Source: CAD feature listing. Evaluate the final solid. Frame: model axes, mm. Face numbers are marked on the shaded views. A direction names the side the tool comes from. Give positions to 0.01 mm unless a question says otherwise; leave off trailing zeros. Write each loop counter-clockwise with the first axis right and the second up, starting at its lowest first coordinate (ties: lowest second). Pieces come first, ordered by that corner, then holes. Notation, with made-up numbers: M 82,-35 L 105,-35 A28 cw 105,3 Z; hole C 9.25,12 d4. An arc over 180 degrees is marked long. Return JSON: item names as keys, results as strings.
Autodesk Inventor part; units mm, degrees
ref_plane "YZ Plane" through (0, 0, 0) normal (1, 0, 0) x (0, 1, 0)
ref_plane "XZ Plane" through (0, 0, 0) normal (0, 1, 0) x (-1, 0, 0)
ref_plane "XY Plane" through (0, 0, 0) normal (0, 0, 1) x (1, 0, 0)
sketch "Sketch1" plane through (0, 0, 0) normal (0, 1, 0) x (-1, 0, 0)
  line L0 (-6.35, 12.7) -> (-6.35, -12.7)
  line L1 (-6.35, -12.7) -> (6.35, -12.7)
  line L2 (6.35, -12.7) -> (6.35, 12.7)
  line L3 (6.35, 12.7) -> (-6.35, 12.7)
  line L4 (-6.35, 12.7) -> (6.35, -12.7) construction
  line L5 (-6.35, -12.7) -> (6.35, 12.7) construction
  line L6 (-6.35, 12.7) -> (19.05, 12.7) construction
  point P0 (0, 0)
  dimension "d0" = 25.4
  dimension "d1" = 90
  dimension "d2" = 12.7
extrude "Baseplate" add sketch "Sketch1" against normal blind 3.175
sketch "Sketch2" plane through (0, -3.175, 0) normal (0, -1, 0) x (1, 0, 0)
  circle A0 centre (3.175, -9.525) radius 1.143
  circle A1 centre (-3.175, 0) radius 1.143
  circle A2 centre (0, 8.5298) radius 1.5
  line L0 (-4.318, -8.382) -> (-2.032, -8.382)
  line L1 (-2.032, -8.382) -> (-2.032, -10.668)
  line L2 (-2.032, -10.668) -> (-4.318, -10.668)
  line L3 (-4.318, -10.668) -> (-4.318, -8.382)
  line L4 (-4.318, -8.382) -> (-2.032, -10.668) construction
  line L5 (-2.032, -8.382) -> (-4.318, -10.668) construction
  point P0 (0, 0)
  point P1 (-3.175, -9.525)
  dimension "d5" = 2.286
  dimension "d6" = 2.286
  dimension "d7" = 3
  dimension "d8" = 2.286
extrude "BoltHole" cut sketch "Sketch2" against normal blind 3.175 contours A2
extrude "Extrusion3" add sketch "Sketch2" along normal blind 3.175 contours A0 | A1 | L0 L1 L2 L3
sketch "Sketch3" plane through (0, -6.35, 0) normal (0, -1, 0) x (1, 0, 0)
  line L0 (-2.032, -11.1125) -> (-4.318, -11.1125)
  line L1 (-4.318, -11.1125) -> (-4.318, -7.9375)
  line L2 (-4.318, -7.9375) -> (-2.032, -7.9375)
  line L3 (-2.032, -7.9375) -> (-2.032, -11.1125)
  line L4 (-2.032, -11.1125) -> (-4.318, -7.9375) construction
  line L5 (-4.318, -11.1125) -> (-2.032, -7.9375) construction
  circle A0 centre (-3.175, 0) radius 1.143
  circle A1 centre (-3.175, 0) radius 1.5875
  circle A2 centre (3.175, -9.525) radius 1.5875
  point P0 (0, 0)
  point P1 (-3.175, -9.525)
  dimension "d13" = 2.286
  dimension "d14" = 3.175
  dimension "d15" = 3.175
  dimension "d16" = 3.175
extrude "Extrusion4" add sketch "Sketch3" along normal blind 1.905 contours L0 L1 L2 L3 | A0 | A1 | A2
chamfer "Chamfer1" distance 1.016 angle 45 4 edges at (-4.7625, -8.255, 0) (1.5875, -8.255, -9.525) (-3.175, -8.255, -7.9375) (-3.175, -8.255, -11.1125)
sketch "Sketch4" plane through (0, -8.255, 0) normal (0, -1, 0) x (1, 0, 0)
  line L0 (5.202, -9.144) -> (1.148, -9.144)
  line L1 (1.148, -9.144) -> (1.148, -9.906)
  line L2 (1.148, -9.906) -> (5.202, -9.906)
  line L3 (5.202, -9.906) -> (5.202, -9.144)
  circle A0 centre (3.175, -9.525) radius 0.5715
  line L4 (5.202, -9.144) -> (1.148, -9.906) construction
  line L5 (1.148, -9.144) -> (5.202, -9.906) construction
  line L6 (-0.7593, 0.381) -> (-5.5907, 0.381)
  line L7 (-5.5907, 0.381) -> (-5.5907, -0.381)
  line L8 (-5.5907, -0.381) -> (-0.7593, -0.381)
  line L9 (-0.7593, -0.381) -> (-0.7593, 0.381)
  line L10 (-0.7593, 0.381) -> (-5.5907, -0.381) construction
  line L11 (-5.5907, 0.381) -> (-0.7593, -0.381) construction
  line L12 (-5.5907, -9.906) -> (-0.7593, -9.906)
  line L13 (-0.7593, -9.906) -> (-0.7593, -9.144)
  line L14 (-0.7593, -9.144) -> (-5.5907, -9.144)
  line L15 (-5.5907, -9.144) -> (-5.5907, -9.906)
  line L16 (-5.5907, -9.906) -> (-0.7593, -9.144) construction
  line L17 (-0.7593, -9.906) -> (-5.5907, -9.144) construction
  point P0 (0, 0)
  point P1 (-3.175, 0)
  point P2 (-3.175, -9.525)
  dimension "d24" = 0.762
  dimension "d25" = 0.762
extrude "Extrusion5" cut sketch "Sketch4" against normal blind 5.08 contours L3 L2 A0 L0 | A0 L2 L0 | A0 L2 L1 L0 | L9 L8 L7 L6 | L15 L14 L13 L12
ref_plane "Work Plane1" through (0, -1.5875, 0) normal (0, 1, 0) x (1, 0, 0)
mirror "Mirror1" about plane through (0, -1.5875, 0) normal (0, 1, 0) of "Extrusion3", "Extrusion4", "Chamfer1", "Extrusion5"
sketch "Sketch5" plane through (0, -3.175, 0) normal (0, -1, 0) x (1, 0, 0)
  line L0 (-6.35, 12.7) -> (-6.35, -12.7)
  line L1 (6.35, 12.7) -> (6.35, -12.7)
  line L2 (-6.35, -12.7) -> (6.35, -12.7)
  line L3 (6.35, -12.7) -> (6.35, 12.7)
  line L4 (6.35, 12.7) -> (-6.35, 12.7)
  line L5 (-6.35, 12.7) -> (-6.35, -12.7)
  point P0 (0, 0)
extrude "Extrusion6" cut sketch "Sketch5" along normal blind 6.0325
properties part number "MirrorBaseplate"
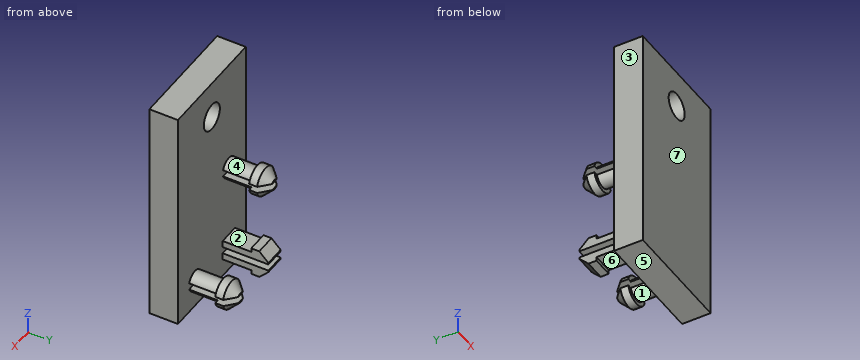
1) Line query: line 1 (Z direction, x = 0, y = -2.45); line 2 (Y direction, x = 3.5, z = 1.5) (3 decimals); line 3 (Z direction, x = -2.25, y = 0.75). Output: solid intervals per line, ascending. Write a range as [from, to].
Numbers:
{"line 1": "z = [-12.7, 7.03], [10.03, 12.7]", "line 2": "y = [-3.175, 0]", "line 3": "z = [-10.67, -9.91], [-9.14, -8.38], [-0.67, -0.38], [0.38, 0.67]"}
2) Cut plane A-A, the plane x = 0. Return the cut outline in (y, z) (3 decimals).
Numbers:
{"outline": "M -3.175,-12.7 L 0,-12.7 L 0,7.03 L -3.175,7.03 Z; M -3.175,10.03 L 0,10.03 L 0,12.7 L -3.175,12.7 Z"}
3) Cut plane D-D, the plane y = -2.25. Return the cut outline in (x, z), then the cut area to 3 significant figures.
Numbers:
{"outline": "M -6.35,-12.7 L 6.35,-12.7 L 6.35,12.7 L -6.35,12.7 Z; hole C 0,8.53 d3", "area": "316 mm²"}
4) Cut plane B-B, the plane y = 2.5. Return the cut outline in (x, z) (3 decimals), then the cut area to 3 significant figures.
Numbers:
{"outline": "M -4.318,-10.668 L -2.032,-10.668 L -2.032,-9.906 L -4.318,-9.906 Z; M -4.318,-9.144 L -2.032,-9.144 L -2.032,-8.382 L -4.318,-8.382 Z; M -4.253,-0.381 A1.143 ccw -2.097,-0.381 Z; M -4.253,0.381 L -2.097,0.381 A1.143 ccw Z; M 2.097,-9.906 A1.143 ccw 4.253,-9.906 Z; M 2.097,-9.144 L 4.253,-9.144 A1.143 ccw Z", "area": "8.27 mm²"}
5) Contact query for flat-ended pins moving along their axis: pin 1 Ø4 at (x, z) = (1.5, -1.5) entering from +Y; pin 2 Ø4 at (x, z) = (-2, 3) entering from +Y; pin 3 Ø1.3 at (y, z) = (3, -8.5) entering from +X; pin 4 Ø2 at (x, y) = (-0.5, 2) entering from +Z. Output: stop coordinate, or through.
Numbers:
{"pin 1": "stops at y = 0", "pin 2": "stops at y = 4.43", "pin 3": "stops at x = 4.71", "pin 4": "passes through"}
6) Cut plane C-C, the plane z = 9.5. Return the cut outline in (x, y) (3 decimals), then the cut area to 3 significant figures.
Numbers:
{"outline": "M -6.35,-3.175 L -1.144,-3.175 L -1.144,0 L -6.35,0 Z; M 1.144,-3.175 L 6.35,-3.175 L 6.35,0 L 1.144,0 Z", "area": "33.1 mm²"}
7) Draft query along Y for the marked faces 5, 6 and 7. Return one class per face: released by +Y, released by -Y, zero draft, split by the parting line, or undercut.
Numbers:
{"face 5": "zero draft", "face 6": "undercut", "face 7": "released by -Y"}
8) Set-up query: the marked faces 1, 2, 3 and 4. Return all of +Z, -Z, +X, -X, +Y, -Y with unobstructed straight access to the full face (end or side cutting, diameter ignored); none if empty.
Numbers:
{"face 1": "-Z", "face 2": "+X, -X", "face 3": "+Z, -Z, -X, +Y, -Y", "face 4": "+Z"}
